from build123d import *

# Parameters (mm, degrees)
SKETCH_W        = 126
SKETCH_H        = 25
SKETCH_R        = 2.2
PAD_DEPTH       = 3
SKETCH001_W     = 12.4
SKETCH001_H     = 4
PAD001_DEPTH    = 21.497
SKETCH002_R     = 2.2
POCKET_DEPTH    = 4
CHAMFER_SIZE    = 1
SKETCH003_R     = 2.65
POCKET001_DEPTH = 24.498
CHAMFER001_SIZE = 1
SKETCH004_R     = 2.65
PAD002_DEPTH    = 1.75


with BuildPart() as part:
    # Sketch → Pad (new body)
    with BuildSketch(Plane.XY):
        Rectangle(SKETCH_W, SKETCH_H)
        with Locations((-53, 0.726)):
            Circle(SKETCH_R, mode=Mode.SUBTRACT)
        with Locations((53, 0.726)):
            Circle(SKETCH_R, mode=Mode.SUBTRACT)
    extrude(amount=PAD_DEPTH)

    # Sketch001 (on Face8 of Pad) → Pad001 (join)
    with BuildSketch(Plane.XY.offset(3)):
        with Locations((-38.154, -3.892)):
            Rectangle(SKETCH001_W, SKETCH001_H)
        with Locations((38.154, -3.892)):
            Rectangle(SKETCH001_W, SKETCH001_H)
    extrude(amount=PAD001_DEPTH)

    # Sketch002 (on Face11 of Pad001) → Pocket (cut)
    with BuildSketch(Plane.XZ.offset(5.892)):
        with Locations((-38.154, 18.297)):
            Circle(SKETCH002_R)
    pocket = extrude(amount=-POCKET_DEPTH, mode=Mode.SUBTRACT)

    # Mirrored: Pocket across Sketch002 V_Axis
    add(pocket.mirror(Plane(origin=(0, -5.892, 0), x_dir=(0, -1, 0), z_dir=(1, 0, 0))), mode=Mode.SUBTRACT)

    # Chamfer
    chamfer_edges = [part.edges().sort_by_distance(p)[0] for p in [
        (0, 12.5, 0),
        (63, 0, 0),
        (0, -12.5, 0),
        (-63, 0, 0),
        (50.8, 0.726, 0),
        (-55.2, 0.726, 0),
    ]]
    chamfer(chamfer_edges, length=CHAMFER_SIZE)

    # Sketch003 (on Face8 of Chamfer) → Pocket001 (cut, through all)
    with BuildSketch(Plane(origin=(0, 0, 0), x_dir=(1, 0, 0), z_dir=(0, 0, -1))):
        with Locations((-38, -4.726)):
            Circle(SKETCH003_R)
        with Locations((-23, -4.726)):
            Circle(SKETCH003_R)
        with Locations((-8, -4.726)):
            Circle(SKETCH003_R)
    extrude(amount=-POCKET001_DEPTH, mode=Mode.SUBTRACT)

    # Chamfer001
    chamfer001_edges = [part.edges().sort_by_distance(p)[0] for p in [
        (-10.65, 4.726, 0),
        (-25.65, 4.726, 0),
        (-40.65, 4.726, 0),
    ]]
    chamfer(chamfer001_edges, length=CHAMFER001_SIZE)

    # Sketch004 (on Face20 of Chamfer001) → Pad002 (join)
    with BuildSketch(Plane.XY.offset(3)):
        with BuildLine():
            ThreePointArc((-38, 8.976), (-42.25, 4.726), (-38, 0.476))
            Line((-38, 0.476), (-8, 0.476))
            ThreePointArc((-8, 0.476), (-3.75, 4.726), (-8, 8.976))
            Line((-38, 8.976), (-8, 8.976))
        make_face()
        with Locations((-38, 4.726)):
            Circle(SKETCH004_R, mode=Mode.SUBTRACT)
        with Locations((-23, 4.726)):
            Circle(SKETCH004_R, mode=Mode.SUBTRACT)
        with Locations((-8, 4.726)):
            Circle(SKETCH004_R, mode=Mode.SUBTRACT)
    extrude(amount=PAD002_DEPTH)


solid = part.part
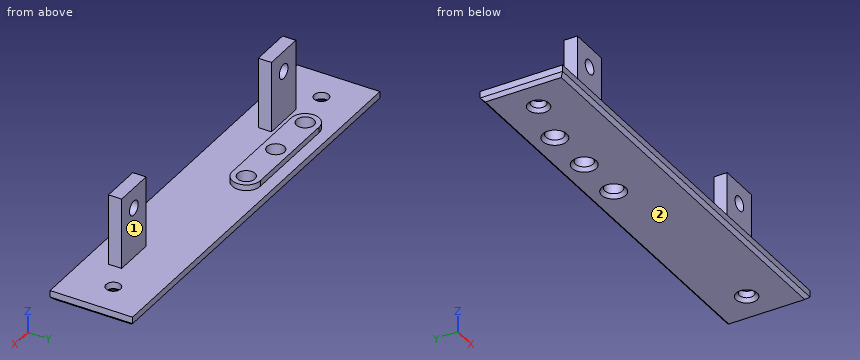
Here's how the part is built. I have some questions about the finished solid (model axes, mm). Face numbers are marked on the shaded views. A direction names the side the tool comes from. Round coordinates to 2 decimals unless told otherwise and drop trailing zeros. Order: outer loops, then holes, each group sorted by start corner. A loop starts at its lowest first (then second) coordinate and runs counter-clockwise, first axis right, second up. Notation, with made-up numbers: (-3.5, -28) -> (49.5, -28) arc R19 ccw to (49.5, -8) -> close; hole circle Ø10 at (87, 64.25). An arc over 180 degrees is marked (long way). Return JSON: item names as keys, results as strings.
Q1. Which directions (+Z, -Z, +X, -X, +Y, -Y) give clear straight access to the entire face, cutting with the end or side of a thin tool? Please do the marked faces 1 and 2.
Filled sheet:
{"face 1": "+Z, +X, -X, +Y", "face 2": "-Z, +X, -X, +Y, -Y"}
Q2. If we section it at C-C on y = 6: Give the number of separate pieces and of enclosed holes in the cut face, plus the area to 3 significant figures.
Filled sheet:
{"separate pieces": "4", "enclosed holes": "0", "area": "374 mm^2"}
Q3. If we section it at D-D on x = 53: List the corners of the cut face in (y, z) for me.
Filled sheet:
{"outline": "(-12.5, 1) -> (-11.5, 0) -> (-2.47, 0) -> (-1.47, 1) -> (-1.47, 3) -> (-12.5, 3) -> close; (2.93, 1) -> (3.93, 0) -> (11.5, 0) -> (12.5, 1) -> (12.5, 3) -> (2.93, 3) -> close"}
Q4. I need wall thicknesses on line 1 along Y through (x, z) = (-23, 2.65); line 2 along X through (y, z) = (-3.5, 13.5); line 3 along Z through (x, y) = (-49.5, 1). Which ranges of each line are inside material? Lowest first, please. Write a range as from..to.
Filled sheet:
{"line 1": "y = -12.5..2.08, 7.38..12.5", "line 2": "x = -44.35..-31.95, 31.95..44.35", "line 3": "z = 0..3"}
Q5. For pin 1 Ø6 at (x, z) = (42.5, 18.5) entering from -Y; pin 2 Ø2.5 at (x, y) = (-21, 4.5) entering from +Z; pin 3 Ø5.5 at (x, y) = (-53, 0.726) entering from -Z; pin 4 Ø2.5 at (x, z) = (38.154, 18.297) entering from +Y, each with a flat end and sliding along its axis, tell me the tip position at first contact or that it passes through.
Filled sheet:
{"pin 1": "stops at y = -5.89", "pin 2": "stops at z = 4.75", "pin 3": "stops at z = 0.45", "pin 4": "passes through"}
Q6. If we section it at B-B on x = -23: List the corners of the cut face in (y, z) for me, plus the area to 3 significant figures.
Filled sheet:
{"outline": "(-12.5, 1) -> (-11.5, 0) -> (1.08, 0) -> (2.08, 1) -> (2.08, 4.75) -> (0.48, 4.75) -> (0.48, 3) -> (-12.5, 3) -> close; (7.38, 1) -> (8.38, 0) -> (11.5, 0) -> (12.5, 1) -> (12.5, 3) -> (8.98, 3) -> (8.98, 4.75) -> (7.38, 4.75) -> close", "area": "62.7 mm^2"}
Q7. If we section it at A-A on z = 23.25: List the corners of the cut face in (x, y) for me, plus the area to 3 significant figures.
Filled sheet:
{"outline": "(-44.35, -5.89) -> (-31.95, -5.89) -> (-31.95, -1.89) -> (-44.35, -1.89) -> close; (31.95, -5.89) -> (44.35, -5.89) -> (44.35, -1.89) -> (31.95, -1.89) -> close", "area": "99.2 mm^2"}
